The listing builds one solid part. Answer for the finished solid, in the listing's coordinates (mm). A direction names the side the tool comes from. Coordinates: 2 decimals unless noted, no trailing zeros. Write each loop counter-clockwise with the first axis right and the second up, starting at its lowest first coordinate (ties: lowest second). Pieces come first, ordered by that corner, then holes.
from build123d import *

# Parameters (mm, degrees)
PAD001_DEPTH    = 10
POCKET002_DEPTH = 76.001
POCKET003_DEPTH = 72.001
FILLET001_R     = 1


with BuildPart() as part:
    # Sketch003 → Pad001 (new body, symmetric)
    with BuildSketch(Plane.XZ):
        with BuildLine():
            Line((5, -18.2), (71, -18.2))
            Line((71, -18.2), (71, -38.2))
            Line((71, -38.2), (76, -38.2))
            Line((76, -38.2), (76, -13.2))
            Line((76, -13.2), (10, -13.2))
            ThreePointArc((5, -8.2), (6.464466, -11.735534), (10, -13.2))
            Line((5, -8.2), (5, 28.2))
            Line((5, 28.2), (0, 28.2))
            Line((0, 28.2), (0, -28.2))
            Line((0, -28.2), (5, -28.2))
            Line((5, -28.2), (5, -18.2))
        make_face()
    extrude(amount=PAD001_DEPTH, both=True)

    # Sketch004 → Pocket002 (cut, through all)
    with BuildSketch(Plane.YZ):
        with BuildLine():
            ThreePointArc((2.2, 22), (0, 24.2), (-2.2, 22))
            Line((-2.2, 22), (-2.2, -2))
            ThreePointArc((-2.2, -2), (0, -4.2), (2.2, -2))
            Line((2.2, 22), (2.2, -2))
        make_face()
    extrude(amount=POCKET002_DEPTH, mode=Mode.SUBTRACT)

    # Sketch005 → Pocket003 (cut, through all)
    with BuildSketch(Plane.YZ.offset(4)):
        with BuildLine():
            ThreePointArc((4.4, 22), (0, 26.4), (-4.4, 22))
            Line((-4.4, -2), (-4.4, 22))
            ThreePointArc((-4.4, -2), (0, -6.4), (4.4, -2))
            Line((4.4, 22), (4.4, -2))
        make_face()
    extrude(amount=POCKET003_DEPTH, mode=Mode.SUBTRACT)

    # Fillet001
    fillet001_edges = [part.edges().sort_by_distance(p)[0] for p in [
        (5, 0, 28.2),
        (2.5, -10, 28.2),
        (2.5, 10, 28.2),
        (2.5, -10, -28.2),
        (2.5, 10, -28.2),
        (73.5, -10, -38.2),
        (73.5, 10, -38.2),
        (76, 0, -38.2),
        (76, 0, -13.2),
        (76, 10, -25.7),
        (76, -10, -25.7),
        (10, 0, -13.2),
        (43, 10, -13.2),
        (43, -10, -13.2),
    ]]
    fillet(fillet001_edges, radius=FILLET001_R)


with BuildPart() as part_1:
    # Body001 placement: moved
    add(part.part.moved(Location((0, 15, 0))))


solid = part_1.part
Q1. The part is cut by section C-C, the plane x = 25. Write down the section's boundary in (y, z), then the cut area to 3 significant figures.
Answers below:
outline: (5, -18.2) - (25, -18.2) - (25, -14.2) arc R1 ccw to (24, -13.2) - (6, -13.2) arc R1 ccw to (5, -14.2) - close
area: 99.6 mm2
Q2. Which of the six approach directions +Z, -Z, +X, -X, +Y, -Y give full straight-line access (tool end or side, diameter ignored) to faces 1 (the face through (5, 15, -23)), 2 (the face through (2, 15, 24.2)), 3 (the face through (4.5, 14.9, -6.4))?
Answers below:
face 1: -Z, +Y, -Y
face 2: +X, -X
face 3: +X
Q3. Determine the mould class of faces 4 (the face through (76, 15, -26)), 5 (the face through (71, 15, -28)), 6 (the face through (2, 12.8, 10)) for opening direction X: released by +X, released by -X, zero draft, split by the parting line, or undercut.
Answers below:
face 4: released by +X
face 5: undercut
face 6: zero draft
Q4. Given pin 1 (1.5 mm diameter, centred on y = 8, z = 5.5, fed in from +X); pin 2 (2.5 mm diameter, centred on x = 2, y = 19, fed in from -Z); pin 3 (7 mm diameter, centred on y = 15.5, z = 8, fed in from +X), each flat-ended and moving along its own axis, determine where each tip first touches the part or whether it passes through.
Answers below:
pin 1: stops at x = 5
pin 2: stops at z = -28.2
pin 3: stops at x = 4
Q5. Find the intervals of material crossed by probe 1 along Z at (x, y) = (17, 7.5); probe 2 along X at (y, z) = (21.25, 8); probe 3 along X at (y, z) = (10.25, -32), in increasing order.
Answers below:
probe 1: z = -18.2 to -13.2
probe 2: x = 0 to 5
probe 3: x = 71 to 76
Q6. The part is cut by section A-A, the plane y = 15. Write down the section's boundary in (x, z).
Answers below:
outline: (0, -28.2) - (5, -28.2) - (5, -18.2) - (71, -18.2) - (71, -38.2) - (75, -38.2) arc R1 ccw to (76, -37.2) - (76, -14.2) arc R1 ccw to (75, -13.2) - (10, -13.2) arc R5 cw to (5, -8.2) - (5, -6.4) - (4, -6.4) - (4, -4.2) - (0, -4.2) - close; (0, 24.2) - (4, 24.2) - (4, 26.4) - (5, 26.4) - (5, 27.2) arc R1 ccw to (4, 28.2) - (0, 28.2) - close
Q7. The part is cut by section B-B, the plane z = 21. Write down the section's boundary in (x, y), then the cut area to 3 significant figures.
Answers below:
outline: (0, 5) - (4, 5) arc R1 ccw to (5, 6) - (5, 10.6) - (4, 10.6) - (4, 12.8) - (0, 12.8) - close; (0, 17.2) - (4, 17.2) - (4, 19.4) - (5, 19.4) - (5, 24) arc R1 ccw to (4, 25) - (0, 25) - close
area: 73.2 mm2
